The listing builds one solid part. Answer for the finished solid, in the listing's coordinates (mm). A direction names the side the tool comes from. Coordinates: 2 decimals unless noted, no trailing zeros. Write each loop counter-clockwise with the first axis right and the second up, starting at its lowest first coordinate (ties: lowest second). Pieces come first, ordered by that corner, then holes.
Autodesk Fusion 360 part; units mm, degrees
sketch "Skizze1" plane through (0, 0, 0) normal (0, 0, 1) x (1, 0, 0) in component "Teigblume"
  circle A0 centre (0, 0) radius 16.5
  dimension "d1" = 33
extrude "Extrusion1" add sketch "Skizze1" along normal blind 25 in component "Teigblume"
fillet "Abrundung1" radius 10 1 edges at (-15.3834, -5.9667, 25) in component "Teigblume"
sketch "Skizze2" plane through (0, 0, 0) normal (0, 1, 0) x (1, 0, 0) in component "Teigblume"
  line L0 (6.5, -17) -> (31.5, -44)
  line L1 (31.5, -44) -> (-31.5, -44)
  line L2 (-31.5, -44) -> (-6.5, -17)
  line L3 (-6.5, -17) -> (6.5, -17)
  line L4 (-16.5, -15) -> (16.5, -15)
  dimension "d6" = 2
  dimension "d7" = 27
  dimension "d8" = 10
  dimension "d9" = 10
  dimension "d19" = 15
  dimension "d20" = 15
extrude "Extrusion2" add sketch "Skizze2" along normal mid plane 10 in component "Teigblume"
fillet "Abrundung2" radius 5 2 edges at (-31.5, 0, 44) (31.5, 0, 44) in component "Teigblume"
fillet "Abrundung3" radius 1 10 edges at (-17.7705, 5, 29.1721) (-24.6379, 5, 41.0018) (0, 5, 44) (24.6379, 5, 41.0018) (17.7705, 5, 29.1721) (17.7705, -5, 29.1721) (24.6379, -5, 41.0018) (0, -5, 44) (-24.6379, -5, 41.0018) (-17.7705, -5, 29.1721) in component "Teigblume"
sketch "Skizze3" plane through (0, 0, 0) normal (0, 0, -1) x (1, 0, 0) in component "Teigblume"
  circle A0 centre (0, 0) radius 16.5
  line L0 (13.2791, 0) -> (6.6395, 11.5)
  line L1 (6.6395, 11.5) -> (-6.6395, 11.5)
  line L2 (-6.6395, 11.5) -> (-13.2791, 0)
  line L3 (-13.2791, 0) -> (-6.6395, -11.5)
  line L4 (-6.6395, -11.5) -> (6.6395, -11.5)
  line L5 (6.6395, -11.5) -> (13.2791, 0)
  dimension "d16" = 11.5
extrude "Extrusion3" cut sketch "Skizze3" against normal blind 13 contours L0 L1 L2 L3 L4 L5 in component "Teigblume"
component "Teigblume" placed x (1, 0, 0) y (0, 1, 0) z (0, 0, 1) at (0, 0, 0)
1. Flat-ended cylindrical pins translate along their axes: P1, Ø16, axis at x = -2, z = 34, coming from the -Y side; P2, Ø0.5, axis at x = 2, y = 6, coming from the +Z side; P3, Ø12, axis at y = -11.5, z = 5, coming from the -X side. Find the tip coordinate at first contact, or state that the pin passes through.
Results found:
P1: stops at y = -5
P2: stops at z = 25
P3: stops at x = -15.56
2. Section A-A on z = 39 is taken. Give the vertices of the cut face in (x, y).
Results found:
outline: (-25.06, -4) arc R1 ccw to (-24.06, -5) - (24.06, -5) arc R1 ccw to (25.06, -4) - (25.06, 4) arc R1 ccw to (24.06, 5) - (-24.06, 5) arc R1 ccw to (-25.06, 4) - close
3. Find the intervals of material crossed by L1, parallel to Y at x = 13, z = 38; L2, parallel to Z at x = -4, y = -2; L3, parallel to Y at x = -6, z = 3.5, in increasing order.
Results found:
L1: y = -5 to 5
L2: z = 13 to 44
L3: y = -15.37 to -11.5, 11.5 to 15.37
4. For a pull along Y with two mould halves and no side action, classify faces 5 (the flat face through (0, 11.5, 6)), 6 (the cylindrical face through (24.67, -0.06, 40.93)), 7 (the cylindrical face through (15.24, 6.32, 7.4)) as pulls with the +Y half, pulls with the -Y half, needs draft (parallel to the pull), parting line crosses it, or undercut.
Results found:
face 5: undercut
face 6: needs draft
face 7: parting line crosses it
5. A tool of negligible diameter and unlimited length cuts with its end or side. For faces 1 (the flat face through (0, 0, 13)), 2 (the flat face through (0, 6, 25)), 3 (the cylindrical face through (17.59, 4.7, 29.4)), 4 (the cylindrical face through (-17.426, 4.699, 29.219)), from which of +Z, -Z, +X, -X, +Y, -Y can it reach the whole face along a straight path? Write none if from no direction.
Results found:
face 1: -Z
face 2: +Z, +X, -X, +Y
face 3: +X, +Y
face 4: -X, +Y
